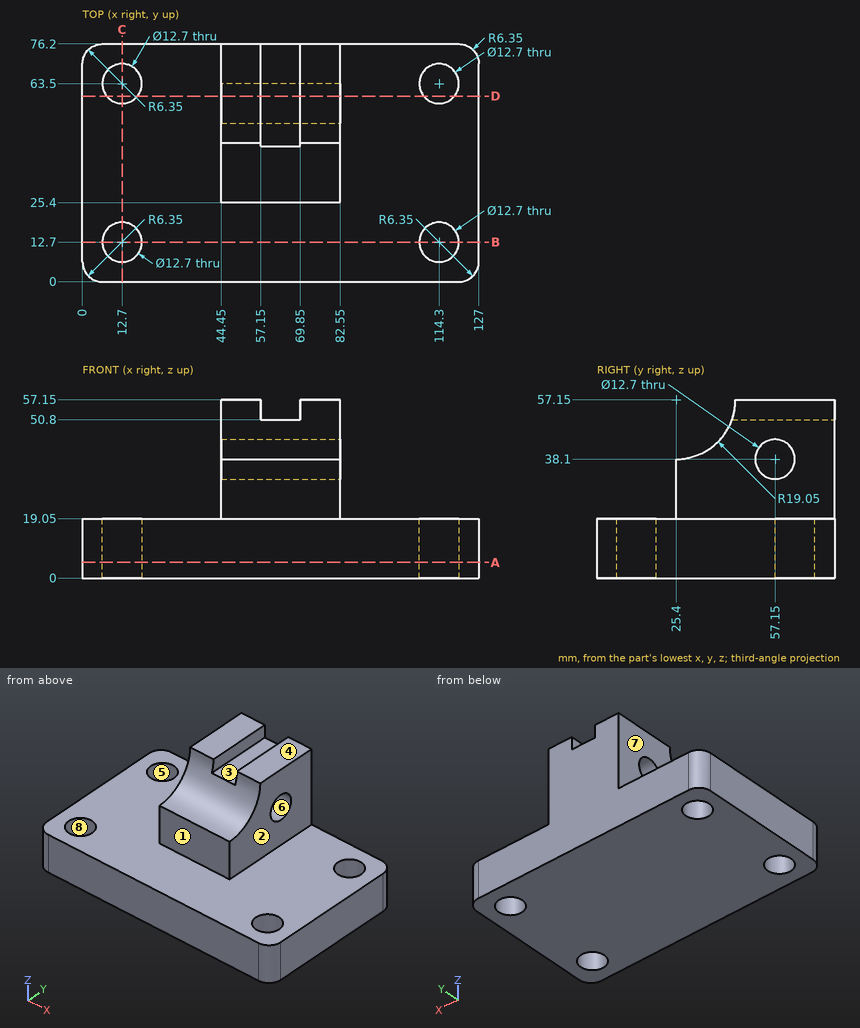
Geometry check sheet. Reference: drawing and pictorial views, mm from the part's lowest x, y, z. A direction names the side the tool comes from. Give positions to 0.01 mm unless a question says otherwise; leave off trailing zeros. Loops run counter-clockwise (first coordinate to the right, second up) from the corner with the lowest first, then second, coordinate; pieces in that order, holes last. Notation, with made-up numbers: (22, 25.25) - (42, 25.25) arc R10 cw to (42, 40.25) - close; hole circle Ø9 at (85.5, 88.25). An arc over 180 degrees is marked (long way). One line per question, with ' | ' between items. Start each with the question number.
1. Cross-section at B-B, the plane y = 12.7. Enter the section's corners in (x, z).
2. Cross-section at C-C, the plane x = 12.7. Enter the section's corners in (y, z), plus the area to 3 significant figures.
3. Draft check along X on the marked faces 5, 6, 7 and 8. Enter one of: released by +X, released by -X, zero draft, split by the parting line, or undercut.
4. Set-up check for the marked faces 1, 2, 3 and 4: record each of +Z, -Z, +X, -X, +Y, -Y from which the full face is reachable in a straight line by a thin tool's end or side.
5. Material ranges on line 1 along Y through (x, z) = (12.7, 4.25); line 2 along Z through (x, y) = (107, 72); line 3 along X through (y, z) = (34, 28), recorded low to high. Write a range as [from, to].
6. Cross-section at D-D, the plane y = 59.5. Enter the section's corners in (x, z), plus the area to 4 significant figures.
7. Cross-section at A-A, the plane z = 5. Enter the section's corners in (x, y).
8. Gauge pin test, flat ends, axial feed: pin 1 Ø21 at (x, z) = (55, 32.5) entering from -Y; pin 2 Ø10 at (y, z) = (59.5, 30.5) entering from +X; pin 3 Ø8 at (y, z) = (24, 40.5) entering from -X. Record the tip position at first contact, or that the pin passes through.
Check result:
1) outline: (0, 0) - (6.35, 0) - (6.35, 19.05) - (0, 19.05) - close; (19.05, 0) - (107.95, 0) - (107.95, 19.05) - (19.05, 19.05) - close; (120.65, 0) - (127, 0) - (127, 19.05) - (120.65, 19.05) - close
2) outline: (0, 0) - (6.35, 0) - (6.35, 19.05) - (0, 19.05) - close; (19.05, 0) - (57.15, 0) - (57.15, 19.05) - (19.05, 19.05) - close; (69.85, 0) - (76.2, 0) - (76.2, 19.05) - (69.85, 19.05) - close | area: 968 mm2
3) face 5: undercut | face 6: zero draft | face 7: released by -X | face 8: undercut
4) face 1: +Z, +X, -X, -Y | face 2: +Z, +X, +Y, -Y | face 3: +Z, +Y, -Y | face 4: +Z, +X, -X, +Y, -Y
5) line 1: y = [0, 6.35], [19.05, 57.15], [69.85, 76.2] | line 2: z = [0, 19.05] | line 3: x = [44.45, 82.55]
6) outline: (0, 0) - (7.77, 0) - (7.77, 19.05) - (0, 19.05) - close; (17.63, 0) - (109.37, 0) - (109.37, 19.05) - (82.55, 19.05) - (82.55, 32.2) - (44.45, 32.2) - (44.45, 19.05) - (17.63, 19.05) - close; (44.45, 44) - (82.55, 44) - (82.55, 57.15) - (69.85, 57.15) - (69.85, 50.8) - (57.15, 50.8) - (57.15, 57.15) - (44.45, 57.15) - close; (119.23, 0) - (127, 0) - (127, 19.05) - (119.23, 19.05) - close | area: 2,965 mm2
7) outline: (0, 6.35) arc R6.35 ccw to (6.35, 0) - (120.65, 0) arc R6.35 ccw to (127, 6.35) - (127, 69.85) arc R6.35 ccw to (120.65, 76.2) - (6.35, 76.2) arc R6.35 ccw to (0, 69.85) - close; hole circle Ø12.7 at (12.7, 12.7); hole circle Ø12.7 at (12.7, 63.5); hole circle Ø12.7 at (114.3, 12.7); hole circle Ø12.7 at (114.3, 63.5)
8) pin 1: stops at y = 25.4 | pin 2: stops at x = 82.55 | pin 3: stops at x = 44.45
